from build123d import *

# Parameters (mm, degrees)
SKETCH_W        = 100
SKETCH_H        = 80
SKETCH_R        = 2
PAD_DEPTH       = 34
SKETCH001_W     = 100
SKETCH001_H     = 80
SKETCH001_R     = 2
PAD001_DEPTH    = 3
CHAMFER_SIZE    = 2
CHAMFER001_SIZE = 2
CHAMFER002_SIZE = 2
CHAMFER003_SIZE = 2
SKETCH004_W     = 8
SKETCH004_H     = 11
SKETCH004_W_2   = 11
SKETCH004_H_2   = 8
PAD002_DEPTH    = 30
POCKET_DEPTH    = 80.001
POCKET001_DEPTH = 100.001
SKETCH005_W     = 4
SKETCH005_H     = 3
POCKET002_DEPTH = 46
SKETCH006_W     = 4
SKETCH006_H     = 3
POCKET003_DEPTH = 45


with BuildPart() as part:
    # Sketch → Pad (new body)
    with BuildSketch(Plane.XY):
        Rectangle(SKETCH_W, SKETCH_H)
        with Locations((-43.75305, -35.00244)):
            Circle(SKETCH_R, mode=Mode.SUBTRACT)
        with Locations((43.75305, 35.00244)):
            Circle(SKETCH_R, mode=Mode.SUBTRACT)
        with Locations((-43.75305, 35.00244)):
            Circle(SKETCH_R, mode=Mode.SUBTRACT)
        with Locations((43.75305, -35.00244)):
            Circle(SKETCH_R, mode=Mode.SUBTRACT)
        Polygon((-47, -26.393398), (-47, 26.393398), (-36.393398, 37), (36.393398, 37), (47, 26.393398), (47, -26.393398), (36.393398, -37), (-36.393398, -37), align=None, mode=Mode.SUBTRACT)
    extrude(amount=PAD_DEPTH)

    # Sketch001 (on Face17 of Pad) → Pad001 (join)
    with BuildSketch(Plane(origin=(0, 0, 0), x_dir=(1, 0, 0), z_dir=(0, 0, -1))):
        Rectangle(SKETCH001_W, SKETCH001_H)
        with Locations((-31.234752, -24.987802)):
            Circle(SKETCH001_R, mode=Mode.SUBTRACT)
        with Locations((31.234752, 24.987802)):
            Circle(SKETCH001_R, mode=Mode.SUBTRACT)
        with Locations((-31.234752, 24.987802)):
            Circle(SKETCH001_R, mode=Mode.SUBTRACT)
        with Locations((31.234752, -24.987802)):
            Circle(SKETCH001_R, mode=Mode.SUBTRACT)
        Polygon((-39.711598, -35.00244), (-41.732324, -31.50244), (-45.773775, -31.50244), (-47.794501, -35.00244), (-45.773775, -38.50244), (-41.732324, -38.50244), align=None, mode=Mode.SUBTRACT)
        Polygon((47.794501, 35.00244), (45.773775, 38.50244), (41.732324, 38.50244), (39.711598, 35.00244), (41.732324, 31.50244), (45.773775, 31.50244), align=None, mode=Mode.SUBTRACT)
        Polygon((-39.711598, 35.00244), (-41.732324, 38.50244), (-45.773775, 38.50244), (-47.794501, 35.00244), (-45.773775, 31.50244), (-41.732324, 31.50244), align=None, mode=Mode.SUBTRACT)
        Polygon((47.794501, -35.00244), (45.773775, -31.50244), (41.732324, -31.50244), (39.711598, -35.00244), (41.732324, -38.50244), (45.773775, -38.50244), align=None, mode=Mode.SUBTRACT)
    extrude(amount=PAD001_DEPTH)

    # Chamfer
    chamfer_edges = [part.edges().sort_by_distance(p)[0] for p in [
        (-33.234752, -24.987802, 0),
    ]]
    chamfer(chamfer_edges, length=CHAMFER_SIZE)

    # Chamfer001
    chamfer001_edges = [part.edges().sort_by_distance(p)[0] for p in [
        (-33.234752, 24.987802, 0),
    ]]
    chamfer(chamfer001_edges, length=CHAMFER001_SIZE)

    # Chamfer002
    chamfer002_edges = [part.edges().sort_by_distance(p)[0] for p in [
        (29.234752, 24.987802, 0),
    ]]
    chamfer(chamfer002_edges, length=CHAMFER002_SIZE)

    # Chamfer003
    chamfer003_edges = [part.edges().sort_by_distance(p)[0] for p in [
        (29.234752, -24.987802, 0),
    ]]
    chamfer(chamfer003_edges, length=CHAMFER003_SIZE)

    # Sketch004 (on Face1 of Chamfer003) → Pad002 (join)
    with BuildSketch(Plane.XY):
        with Locations((-15, -34.5)):
            Rectangle(SKETCH004_W, SKETCH004_H)
        with Locations((15, 34.5)):
            Rectangle(SKETCH004_W, SKETCH004_H)
        with Locations((15, -34.5)):
            Rectangle(SKETCH004_W, SKETCH004_H)
        with Locations((-15, 34.5)):
            Rectangle(SKETCH004_W, SKETCH004_H)
        with Locations((-44.5, 15)):
            Rectangle(SKETCH004_W_2, SKETCH004_H_2)
        with Locations((44.5, 15)):
            Rectangle(SKETCH004_W_2, SKETCH004_H_2)
        with Locations((44.5, -15)):
            Rectangle(SKETCH004_W_2, SKETCH004_H_2)
        with Locations((-44.5, -15)):
            Rectangle(SKETCH004_W_2, SKETCH004_H_2)
    extrude(amount=PAD002_DEPTH)

    # Sketch002 (on Face85 of Pad002) → Pocket (cut, through all)
    with BuildSketch(Plane.XZ.offset(40)):
        with BuildLine():
            Line((-19, 34), (-19, 30))
            ThreePointArc((-19, 30), (-15, 26), (-11, 30))
            Line((-11, 34), (-11, 30))
            Line((-11, 34), (-19, 34))
        make_face()
        with BuildLine():
            Line((19, 34), (19, 30))
            ThreePointArc((11, 30), (15, 26), (19, 30))
            Line((11, 34), (11, 30))
            Line((11, 34), (19, 34))
        make_face()
    extrude(amount=-POCKET_DEPTH, mode=Mode.SUBTRACT)

    # Sketch003 (on Face108 of Pocket) → Pocket001 (cut, through all)
    with BuildSketch(Plane(origin=(-50, 0, 0), x_dir=(0, -1, 0), z_dir=(-1, 0, 0))):
        with BuildLine():
            Line((-19, 34), (-19, 30))
            ThreePointArc((-19, 30), (-15, 26), (-11, 30))
            Line((-11, 34), (-11, 30))
            Line((-11, 34), (-19, 34))
        make_face()
        with BuildLine():
            Line((19, 34), (19, 30))
            ThreePointArc((11, 30), (15, 26), (19, 30))
            Line((11, 34), (11, 30))
            Line((11, 34), (19, 34))
        make_face()
    extrude(amount=-POCKET001_DEPTH, mode=Mode.SUBTRACT)

    # Sketch005 (on Face24 of Pocket001) → Pocket002 (cut)
    with BuildSketch(Plane.XZ.offset(19)):
        with Locations((-43, 21.5)):
            Rectangle(SKETCH005_W, SKETCH005_H)
        with Locations((43, 21.5)):
            Rectangle(SKETCH005_W, SKETCH005_H)
    extrude(amount=-POCKET002_DEPTH, mode=Mode.SUBTRACT)

    # Sketch006 (on Face12 of Pocket002) → Pocket003 (cut)
    with BuildSketch(Plane(origin=(-19, 0, 0), x_dir=(0, -1, 0), z_dir=(-1, 0, 0))):
        with Locations((-33, 21.5)):
            Rectangle(SKETCH006_W, SKETCH006_H)
        with Locations((33, 21.5)):
            Rectangle(SKETCH006_W, SKETCH006_H)
    extrude(amount=-POCKET003_DEPTH, mode=Mode.SUBTRACT)


solid = part.part
Model file for the job. Use its own axes, mm. A direction names the side the tool comes from. Coordinates: 2 decimals unless noted, no trailing zeros. Write each loop counter-clockwise with the first axis right and the second up, starting at its lowest first coordinate (ties: lowest second). Pieces come first, ordered by that corner, then holes. Notation, with made-up numbers: (-21, 74.25) -> (6, 74.25) arc R23 ccw to (6, 85.25) -> close; hole circle Ø11 at (-19.75, 35.5). An arc over 180 degrees is marked (long way). One line per item, written item: value. Start each with the question number.
1) Slice it at D-D on y = -5.5. Write the cut outline in (x, z).
2) Slice it at B-B on x = 15. Write the cut outline in (y, z), then the cut area to 3 significant figures.
3) Pull direction Y, two halves, no side cores. Call faces 5 (the face through (43, 15, 20)), 6 (the face through (11, -39, 32)): +Y half, -Y half, draft (parallel to the pull), parting line (faces both ways), or undercut.
4) Slice it at A-A on y = 15. Write the cut outline in (x, z), then the cut area to 3 significant figures.
5) Which spindle directions (+Z, -Z, +X, -X, +Y, -Y) get a long thin tool onto all of the face, cutting with end or side? Do faces 1 (the face through (15, 33, 23)), 2 (the face through (-46.77, 33.23, -1.48)), 3 (the face through (39, -15, 15)), 4 (the face through (40, -35, 34)). Say none if no direction does.
6) Slice it at C-C on x = 1. Write the cut outline in (y, z), then the cut area to 3 significant figures.
7) Flat gauge pins, fed straight in: pin 1 Ø3 at (x, y) = (-5, -9.5) entering from +Z; pin 2 Ø2.5 at (x, y) = (-31.23, -24.99) entering from -Z; pin 3 Ø1.2 at (x, y) = (-14.5, -33) entering from +Z; pin 4 Ø2 at (x, y) = (14.5, -33.5) entering from +Z. Where does each tip first touch, or does it go through?
8) Probe probe 1 along Y at (x, z) = (-1, 29); probe 2 along X at (y, z) = (22, 4.5); probe 3 along Y at (x, z) = (41.5, 4). List the from-to ranges inside material, lowest first.
Answers follow:
1. outline: (-50, -3) -> (50, -3) -> (50, 34) -> (47, 34) -> (47, 0) -> (-47, 0) -> (-47, 34) -> (-50, 34) -> close
2. outline: (-40, -3) -> (40, -3) -> (40, 26) -> (29, 26) -> (29, 0) -> (-29, 0) -> (-29, 26) -> (-40, 26) -> close; hole (-35, 20) -> (-31, 20) -> (-31, 23) -> (-35, 23) -> close; hole (31, 20) -> (35, 20) -> (35, 23) -> (31, 23) -> close
2. area: 788 mm2
3. face 5: undercut
3. face 6: draft
4. outline: (-50, -3) -> (50, -3) -> (50, 26) -> (39, 26) -> (39, 0) -> (-39, 0) -> (-39, 26) -> (-50, 26) -> close; hole (-45, 20) -> (-41, 20) -> (-41, 23) -> (-45, 23) -> close; hole (41, 20) -> (45, 20) -> (45, 23) -> (41, 23) -> close
4. area: 848 mm2
5. face 1: none
5. face 2: -Z
5. face 3: +Z
5. face 4: +Z, +X, -X, +Y, -Y
6. outline: (-40, -3) -> (40, -3) -> (40, 34) -> (37, 34) -> (37, 0) -> (-37, 0) -> (-37, 34) -> (-40, 34) -> close
6. area: 444 mm2
7. pin 1: z = 0
7. pin 2: through
7. pin 3: z = 26.15
7. pin 4: z = 26.29
8. probe 1: -40 to -37, 37 to 40
8. probe 2: -50 to -47, 47 to 50
8. probe 3: -40 to -31.89, -19 to -11, 11 to 19, 31.89 to 40
